Autodesk Inventor part; units mm, degrees
ref_plane "YZ Plane" through (0, 0, 0) normal (1, 0, 0) x (0, 1, 0)
ref_plane "XZ Plane" through (0, 0, 0) normal (0, 1, 0) x (-1, 0, 0)
ref_plane "XY Plane" through (0, 0, 0) normal (0, 0, 1) x (1, 0, 0)
sketch "Sketch1" plane through (0, 0, 0) normal (0, 1, 0) x (-1, 0, 0)
  line L0 (-150, -150) -> (150, -150)
  line L1 (150, -150) -> (150, 150)
  line L2 (150, 150) -> (-150, 150)
  line L3 (-150, 150) -> (-150, -150)
  line L4 (-150, -150) -> (150, 150) construction
  line L5 (150, -150) -> (-150, 150) construction
  point P0 (0, 0)
extrude "Extrusion1" add sketch "Sketch1" along normal blind 40
sketch "Sketch4" plane through (0, 0, 0) normal (0, -1, 0) x (1, 0, 0)
  line L0 (150, -150) -> (-150, -150)
  line L1 (0, -150) -> (150, -150)
  line L2 (60, -130) -> (90, -130)
  line L3 (90, -130) -> (90, -140)
  line L4 (90, -140) -> (60, -140)
  line L5 (60, -140) -> (60, -130)
  line L6 (60, -130) -> (90, -140) construction
  line L7 (90, -130) -> (60, -140) construction
  line L8 (-60, -130) -> (-90, -130)
  line L9 (-90, -130) -> (-90, -140)
  line L10 (-90, -140) -> (-60, -140)
  line L11 (-60, -140) -> (-60, -130)
  line L12 (150, 150) -> (150, -150)
  line L13 (60, 130) -> (90, 130)
  line L14 (90, 130) -> (90, 140)
  line L15 (90, 140) -> (60, 140)
  line L16 (60, 140) -> (60, 130)
  line L17 (60, 130) -> (90, 140) construction
  line L18 (90, 130) -> (60, 140) construction
  line L19 (-60, 130) -> (-90, 130)
  line L20 (-60, 140) -> (-60, 130)
  line L21 (-90, 140) -> (-60, 140)
  line L22 (-90, 130) -> (-90, 140)
  point P0 (0, 0)
extrude "Extrusion3" add sketch "Sketch4" along normal blind 30
sketch "Sketch5" plane through (0, 0, 0) normal (0, -1, 0) x (1, 0, 0)
  line L0 (-40, 22.5) -> (-50, 22.5)
  line L1 (-50, 22.5) -> (-50, -22.5)
  line L2 (-50, -22.5) -> (-40, -22.5)
  line L3 (-40, -22.5) -> (-40, 22.5)
  line L4 (-40, 22.5) -> (-50, -22.5) construction
  line L5 (-50, 22.5) -> (-40, -22.5) construction
  line L6 (-16, -22.5) -> (-6, -22.5)
  line L7 (-6, -22.5) -> (-6, 22.5)
  line L8 (-6, 22.5) -> (-16, 22.5)
  line L9 (-16, 22.5) -> (-16, -22.5)
  line L10 (40, 22.5) -> (50, 22.5)
  line L11 (50, 22.5) -> (50, -22.5)
  line L12 (50, -22.5) -> (40, -22.5)
  line L13 (40, -22.5) -> (40, 22.5)
  line L14 (40, 22.5) -> (50, -22.5) construction
  line L15 (50, 22.5) -> (40, -22.5) construction
  line L16 (16, -22.5) -> (6, -22.5)
  line L17 (6, -22.5) -> (6, 22.5)
  line L18 (6, 22.5) -> (16, 22.5)
  line L19 (16, 22.5) -> (16, -22.5)
  point P0 (0, 0)
  point P1 (-45, 0)
  point P2 (45, 0)
extrude "Extrusion4" add sketch "Sketch5" along normal blind 30
sketch "Sketch6" plane through (40, 0, -22.5) normal (-1, 0, 0) x (0, 0, 1)
  line L0 (0, 0) -> (0, -30)
  line L1 (45, -30) -> (0, -30)
  line L2 (0, -30) -> (0, -24)
  line L3 (0, -24) -> (45, -24)
  line L4 (45, -24) -> (45, -30)
  point P0 (22.5, 0)
extrude "Extrusion5" add sketch "Sketch6" along normal blind 24
sketch "Sketch9" plane through (-40, 0, 22.5) normal (1, 0, 0) x (0, 0, -1)
  line L0 (0, 0) -> (0, -30)
  line L1 (45, -30) -> (0, -30)
  line L2 (0, -30) -> (0, -24)
  line L3 (0, -24) -> (45, -24)
  line L4 (45, -24) -> (45, -30)
  point P0 (22.5, 0)
extrude "Extrusion6" add sketch "Sketch9" along normal blind 24
sketch "Sketch12" plane through (0, 0, 0) normal (0, -1, 0) x (1, 0, 0)
  circle A0 centre (-40, -37.5) radius 2.5
  circle A1 centre (-16, -37.5) radius 2.5
  line L0 (0, 0) -> (11, 0)
  circle A2 centre (16, 37.5) radius 2.5
  circle A3 centre (40, 37.5) radius 2.5
hole "Hole1" at (-40, 0, -37.5) at (-16, 0, -37.5) at (16, 0, 37.5) at (40, 0, 37.5) direction (0, 1, 0) diameter 5 end through all
sketch "Sketch14" plane through (0, 40, 0) normal (0, 1, 0) x (1, 0, 0)
  line L0 (150, -150) -> (150, 150)
  line L1 (150, 0) -> (150, 34.3)
  line L2 (130, 33.8503) -> (130, 43.8503)
  line L3 (130, 43.8503) -> (56.6, 43.8503)
  line L4 (56.6, 43.8503) -> (56.6, -42.9497)
  line L5 (56.6, -42.9497) -> (130, -42.9497)
  line L6 (130, -42.9497) -> (130, 43.8503)
  line L7 (66.6, 43.8503) -> (56.6, 43.8503)
  line L8 (130, 53.8503) -> (140, 53.8503)
  line L9 (140, 53.8503) -> (46.6, 53.8503)
  line L10 (46.6, 53.8503) -> (46.6, -54.1497)
  line L11 (46.6, -54.1497) -> (140, -54.1497)
  line L12 (140, -54.1497) -> (140, 53.8503)
  point P0 (0, 0)
extrude "Extrusion10" add sketch "Sketch14" along normal blind 20
sketch "Sketch17" plane through (0, -30, 0) normal (0, -1, 0) x (1, 0, 0)
  line L0 (-90, 130) -> (-60, 130)
  line L1 (-60, 130) -> (-60, 140)
  line L2 (-60, 140) -> (-90, 140)
  line L3 (-90, 140) -> (-90, 130)
  point P0 (0, 0)
sketch "Sketch18" plane through (0, -30, 0) normal (0, -1, 0) x (1, 0, 0)
  line L0 (60, 130) -> (90, 130)
  line L1 (90, 130) -> (90, 140)
  line L2 (90, 140) -> (60, 140)
  line L3 (60, 140) -> (60, 130)
  point P0 (0, 0)
sketch "Sketch19" plane through (0, -30, 0) normal (0, -1, 0) x (1, 0, 0)
  line L0 (-60, -130) -> (-90, -130)
  line L1 (-90, -130) -> (-90, -140)
  line L2 (-90, -140) -> (-60, -140)
  line L3 (-60, -140) -> (-60, -130)
  point P0 (0, 0)
sketch "Sketch20" plane through (0, -30, 0) normal (0, -1, 0) x (1, 0, 0)
  line L0 (90, -130) -> (60, -130)
  line L1 (60, -130) -> (60, -140)
  line L2 (60, -140) -> (90, -140)
  line L3 (90, -140) -> (90, -130)
  point P0 (0, 0)
extrude "Extrusion11" add sketch "Sketch17" along normal blind 50
extrude "Extrusion12" add sketch "Sketch19" along normal blind 50
extrude "Extrusion13" add sketch "Sketch20" along normal blind 50
extrude "Extrusion14" add sketch "Sketch18" along normal blind 50
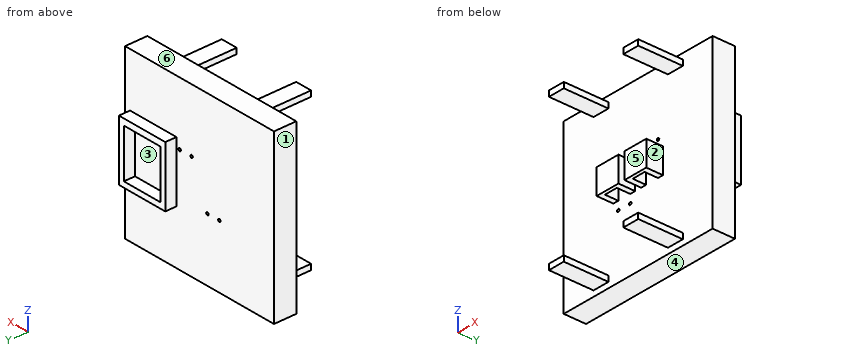
Model file for the job. Use its own axes, mm. Face numbers are marked on the shaded views. A direction names the side the tool comes from. Round coordinates to 2 decimals unless told otherwise and drop trailing zeros. Loops run counter-clockwise (first coordinate to the right, second up) from the corner with the lowest first, then second, coordinate; pieces in that order, holes last. Notation, with made-up numbers: (-30, -14) -> (13, -14) arc R18 cw to (13, 12) -> close; hole circle Ø2 at (0, -15). An arc over 180 degrees is marked (long way). Answer as CSV lines item,"result". Start each with the question number.
1) Mould opens along Z. For the marked faces 3, 4, 5 and 6 say: +Z half, -Z half, draft (parallel to the pull), parting line (faces both ways), or undercut.
2) Probe line 1 along X through (y, z) = (9, 37.5); line 2 along X through (y, z) = (44.5, -7.5); line 3 along Z through (x, y) = (16, 24). List the from-to ranges inside material, lowest first.
3) Pin check, flat tips, straight feed: P1, Ø7, axis at x = -24, z = -7, coming from the +Y side; P2, Ø19, axis at y = -10.5, z = -7.5, coming from the +X side; P3, Ø12, axis at x = 85, z = -26.5, coming from the -Y side; P4, Ø22, axis at y = 50.5, z = -13.5, coming from the +X side. Stop position of each tip, or through.
4) Tool access for the marked faces 1 and 2: list every direction of +Z, -Z, +X, -X, +Y, -Y with a clear straight run to the whole face (end or side of a thin tool).
5) Slice it at D-D (x = -125). List the corners of the cut face in (y, z), plus the area to 3 significant figures.
6) Slice it at B-B (z = 6). List the corners of the cut face in (x, y).
7) Slice it at A-A (y = -38). List the corners of the cut face in (x, z), plus the area to 3 significant figures.
8) Slice it at C-C (y = 51). List the corners of the cut face in (x, z).
Filled in:
1,face 3,"undercut"
1,face 4,"-Z half"
1,face 5,"draft"
1,face 6,"+Z half"
2,line 1,"x = -150 to 13.5, 18.5 to 37.5, 42.5 to 150"
2,line 2,"x = 46.6 to 56.6, 130 to 140"
2,line 3,"z = -150 to 35, 40 to 150"
3,P1,"stops at y = 40"
3,P2,"stops at x = 50"
3,P3,"stops at y = 0"
3,P4,"stops at x = 150"
4,face 1,"+Z, -Z, -X, +Y, -Y"
4,face 2,"+Z, -Z, +X, -Y"
5,outline,"(0, -150) -> (40, -150) -> (40, 150) -> (0, 150) -> close"
5,area,"12,000 mm2"
6,outline,"(-150, 0) -> (-50, 0) -> (-50, -30) -> (-6, -30) -> (-6, 0) -> (6, 0) -> (6, -30) -> (50, -30) -> (50, 0) -> (150, 0) -> (150, 40) -> (140, 40) -> (140, 60) -> (130, 60) -> (130, 40) -> (56.6, 40) -> (56.6, 60) -> (46.6, 60) -> (46.6, 40) -> (-150, 40) -> close; hole (-40, -24) -> (-16, -24) -> (-16, 0) -> (-40, 0) -> close; hole (16, -24) -> (40, -24) -> (40, 0) -> (16, 0) -> close"
7,outline,"(-90, -140) -> (-60, -140) -> (-60, -130) -> (-90, -130) -> close; (-90, 130) -> (-60, 130) -> (-60, 140) -> (-90, 140) -> close; (60, -140) -> (90, -140) -> (90, -130) -> (60, -130) -> close; (60, 130) -> (90, 130) -> (90, 140) -> (60, 140) -> close"
7,area,"1,200 mm2"
8,outline,"(46.6, -53.85) -> (140, -53.85) -> (140, 54.15) -> (46.6, 54.15) -> close; hole (56.6, -43.85) -> (130, -43.85) -> (130, 42.95) -> (56.6, 42.95) -> close"
